```python
from build123d import *

# Parameters (mm, degrees)
SKETCH_1_R                  = 2.25
SKETCH_1_R_2                = 4
EXTRUDE_1_DEPTH             = 2
SKETCH_3_R                  = 0.55
CUT_EXTRUDE_1_DEPTH         = 2
PATTERN_LINEAR_1_COUNT      = 2
PATTERN_LINEAR_1_PITCH      = 2
PATTERN_LINEAR_1_COUNT_DIR2 = 12
PATTERN_LINEAR_1_PITCH_DIR2 = 2.54
SKETCH_4_R                  = 0.9
CUT_EXTRUDE_2_DEPTH         = 2
SKETCH_5_R                  = 0.9
CUT_EXTRUDE_3_DEPTH         = 10
SKETCH_6_R                  = 7.5
SKETCH_6_R_2                = 2.5
SKETCH_6_W                  = 15
SKETCH_6_H                  = 28
SKETCH_6_W_2                = 29
SKETCH_6_H_2                = 5
EXTRUDE_2_DEPTH             = 10
SKETCH_7_W                  = 15
SKETCH_7_H                  = 28
EXTRUDE_3_DEPTH             = 15
SKETCH_8_R                  = 2.5
EXTRUDE_4_DEPTH             = 15.5
SKETCH_9_R                  = 3
EXTRUDE_5_DEPTH             = 5
SKETCH_10_R                 = 3
SKETCH_10_R_2               = 0.3
CUT_EXTRUDE_4_DEPTH         = 4.5
CHAMFER_1_SIZE              = 0.5


with BuildPart() as part:
    # Эскиз1 → Вытянуть1 (new body)
    with BuildSketch(Plane.XY):
        Polygon((10, -60), (65, -60), (65, 60), (-95, 60), (-95, -60), (-20, -60), (-20, -30), (10, -30), align=None)
        with Locations((-90, 55)):
            Circle(SKETCH_1_R, mode=Mode.SUBTRACT)
        with Locations((60, 55)):
            Circle(SKETCH_1_R, mode=Mode.SUBTRACT)
        with Locations((60, -55)):
            Circle(SKETCH_1_R, mode=Mode.SUBTRACT)
        with Locations((-90, -55)):
            Circle(SKETCH_1_R, mode=Mode.SUBTRACT)
        with Locations((-60, 22)):
            Circle(SKETCH_1_R_2, mode=Mode.SUBTRACT)
        with Locations((-30.5, 22)):
            Circle(SKETCH_1_R_2, mode=Mode.SUBTRACT)
        with Locations((-30.5, -23)):
            Circle(SKETCH_1_R_2, mode=Mode.SUBTRACT)
        with Locations((-60, -23)):
            Circle(SKETCH_1_R_2, mode=Mode.SUBTRACT)
        with Locations((24.25, -22.5)):
            Circle(SKETCH_1_R_2, mode=Mode.SUBTRACT)
    extrude(amount=EXTRUDE_1_DEPTH)

    # Эскиз3 → Вырез-Вытянуть1 (cut)
    with BuildSketch(Plane.XY.offset(2)):
        with Locations((-2.25, 7.75)):
            Circle(SKETCH_3_R)
    cut_extrude_1 = extrude(amount=-CUT_EXTRUDE_1_DEPTH, mode=Mode.SUBTRACT)

    # Линейный массив1: Cut-Extrude 1 2 × 12
    with Locations(*[(i * PATTERN_LINEAR_1_PITCH, -j * PATTERN_LINEAR_1_PITCH_DIR2, 0) for i in range(PATTERN_LINEAR_1_COUNT) for j in range(PATTERN_LINEAR_1_COUNT_DIR2) if (i, j) != (0, 0)]):
        add(cut_extrude_1, mode=Mode.SUBTRACT)

    # Эскиз4 → Вырез-Вытянуть2 (cut)
    with BuildSketch(Plane.XY.offset(2)):
        with Locations((17.75, -46.75)):
            Circle(SKETCH_4_R)
        with Locations((-24.75, 16.23)):
            Circle(SKETCH_4_R)
        with Locations((-88.25, 1.58)):
            Circle(SKETCH_4_R)
        with Locations((18, -41.5)):
            Circle(SKETCH_4_R)
        with Locations((14.5, -23.5)):
            Circle(SKETCH_4_R)
        with Locations((18, -36.42)):
            Circle(SKETCH_4_R)
        with Locations((-22.75, 16.23)):
            Circle(SKETCH_4_R)
        with Locations((-4.75, 16.23)):
            Circle(SKETCH_4_R)
        with Locations((18, -31.34)):
            Circle(SKETCH_4_R)
        with Locations((-88.25, -3.5)):
            Circle(SKETCH_4_R)
    extrude(amount=-CUT_EXTRUDE_2_DEPTH, mode=Mode.SUBTRACT)

    # Эскиз5 → Вырез-Вытянуть3 (cut)
    with BuildSketch(Plane.XY.offset(2)):
        with Locations((41.75, 35.75)):
            Circle(SKETCH_5_R)
        with Locations((51.75, 35.75)):
            Circle(SKETCH_5_R)
        with Locations((6.75, 42)):
            Circle(SKETCH_5_R)
        with Locations((16.75, 42)):
            Circle(SKETCH_5_R)
        with Locations((41.75, -35.5)):
            Circle(SKETCH_5_R)
        with Locations((51.75, -35.5)):
            Circle(SKETCH_5_R)
        with Locations((41.75, 0.25)):
            Circle(SKETCH_5_R)
        with Locations((51.75, 0.25)):
            Circle(SKETCH_5_R)
        with Locations((12.25, -55)):
            Circle(SKETCH_5_R)
        with Locations((-79, 56.25)):
            Circle(SKETCH_5_R)
        with Locations(Location((-79, -56.5, 0), (0, 0, 180))):
            Circle(SKETCH_5_R)
        with Locations((8.75, 18.5)):
            Circle(SKETCH_5_R)
        with Locations((16.5, -8)):
            Circle(SKETCH_5_R)
        with Locations((7.75, -22.5)):
            Circle(SKETCH_5_R)
    extrude(amount=-CUT_EXTRUDE_3_DEPTH, mode=Mode.SUBTRACT)

    # Эскиз6 → Вытянуть2 (add)
    # profile 1 of 4: a face of its own
    with BuildSketch(Plane.XY.offset(2)):
        with Locations(Location((-14.5, 1.75, 0), (0, 0, 180))):
            Circle(SKETCH_6_R)
        with Locations((-14.5, 1.75)):
            Circle(SKETCH_6_R_2, mode=Mode.SUBTRACT)
    # profile 2 of 4: a face of its own
    with BuildSketch(Plane.XY.offset(2)):
        with Locations((-69.2, 0)):
            Rectangle(SKETCH_6_W, SKETCH_6_H)
    # profile 3 of 4: a face of its own
    with BuildSketch(Plane.XY.offset(2)):
        with Locations((-41.5, 6.5)):
            Rectangle(SKETCH_6_W_2, SKETCH_6_H_2)
    # profile 4 of 4: a face of its own
    with BuildSketch(Plane.XY.offset(2)):
        with Locations((-41.5, -8.5)):
            Rectangle(SKETCH_6_W_2, SKETCH_6_H_2)
    extrude(amount=EXTRUDE_2_DEPTH)

    # Эскиз7 → Вытянуть3 (add)
    with BuildSketch(Plane.XY.offset(12)):
        with Locations((-69.2, 0)):
            Rectangle(SKETCH_7_W, SKETCH_7_H)
    extrude(amount=EXTRUDE_3_DEPTH)

    # Эскиз8 → Вытянуть4 (add)
    with BuildSketch(Plane.XY.offset(2)):
        with Locations((-8.5, -18)):
            Circle(SKETCH_8_R)
    extrude(amount=-EXTRUDE_4_DEPTH)

    # Эскиз9 → Вытянуть5 (add)
    with BuildSketch(Plane(origin=(0, 0, 0), x_dir=(-1, 0, 0), z_dir=(0, 0, -1))):
        with Locations((8.5, -18)):
            Circle(SKETCH_9_R)
    extrude(amount=EXTRUDE_5_DEPTH)

    # Эскиз10 → Вырез-Вытянуть4 (cut)
    with BuildSketch(Plane.XY):
        with Locations((-8.5, -18)):
            Circle(SKETCH_10_R)
        with Locations((-8.5, -16.496281754)):
            Circle(SKETCH_10_R_2, mode=Mode.SUBTRACT)
        with Locations((-9.77, -19.036281754)):
            Circle(SKETCH_10_R_2, mode=Mode.SUBTRACT)
        with Locations((-7.23, -19.036281754)):
            Circle(SKETCH_10_R_2, mode=Mode.SUBTRACT)
    extrude(amount=-CUT_EXTRUDE_4_DEPTH, mode=Mode.SUBTRACT)

    # Фаска1
    chamfer_1_edges = [part.edges().sort_by_distance(p)[0] for p in [
        (-11, -18, -13.5),
    ]]
    chamfer(chamfer_1_edges, length=CHAMFER_1_SIZE)


solid = part.part
```
The model under review builds one solid part; all positions refer to its coordinate system, in mm. A direction names the side the tool comes from. Coordinates: 2 decimals unless noted, no trailing zeros. Write each loop counter-clockwise with the first axis right and the second up, starting at its lowest first coordinate (ties: lowest second). Pieces come first, ordered by that corner, then holes. Notation, with made-up numbers: (-4, 34.5) - (16, 34.5) arc R16 cw to (16, 42.5) - close; hole circle Ø7 at (54.25, 66.5). An arc over 180 degrees is marked (long way). Write item = value, one per line.
(1) For P1, Ø1.8, axis at x = -0.25, y = -10.03, coming from the -Z side; P2, Ø1.5, axis at y = 6.5, z = 4.5, coming from the -X side; P3, Ø6, axis at x = -90, y = 55, coming from the +Z side, all flat-tipped, find the tip position at first contact; note any pin that passes through.
Result sheet:
P1 = 0
P2 = -76.7
P3 = 2
(2) Machinability: for faces 5 (the face through (-42, -11, 7)), 6 (the face through (-27, 6, 7)), 7 (the face through (-69, 14, 14)), 8 (the face through (-42, 4, 7)), which of the approach directions +Z, -Z, +X, -X, +Y, -Y give a long, thin tool a straight path to every point of the face, cutting with its end or side? Answer none if there is none.
Result sheet:
face_5 = +Z, +X, -Y
face_6 = +Z, +Y, -Y
face_7 = +Z, +X, -X, +Y
face_8 = +Z
(3) For line 1 (Y direction, x = -30, z = 1); line 2 (X direction, y = -46.75, z = 1); line 3 (X direction, y = 42, z = 1), list the stretches that pass through material, from the lowest coordinate up. Write a range as [from, to].
Result sheet:
line_1 = [-60, -26.97], [-19.03, 18.03], [25.97, 60]
line_2 = [-95, -20], [10, 16.85], [18.65, 65]
line_3 = [-95, 5.85], [7.65, 15.85], [17.65, 65]
(4) Mouldability with a two-part tool opening along X and no side actions: class faces 1 (the face through (-56, -9, 7)), 2 (the face through (-27, -9, 7)), 3 (the face through (-9.884, -20.662, -4.746)), 4 (the face through (-42, -8, 12)) as pulls with the +X half, pulls with the -X half, needs draft (parallel to the pull), parting line crosses it, or undercut.
Result sheet:
face_1 = undercut
face_2 = pulls with the +X half
face_3 = parting line crosses it
face_4 = needs draft
(5) Consider section A-A, the plane z = 6. Give the boundary of the cut face in (x, y).
Result sheet:
outline = (-76.7, -14) - (-61.7, -14) - (-61.7, 14) - (-76.7, 14) - close; (-56, -11) - (-27, -11) - (-27, -6) - (-56, -6) - close; (-56, 4) - (-27, 4) - (-27, 9) - (-56, 9) - close; circle Ø15 at (-14.5, 1.75); hole circle Ø5 at (-14.5, 1.75)
(6) Consider section C-C, the plane x = -51. Give the boundary of the cut face in (y, z), then the cut area to 3 significant figures.
Result sheet:
outline = (-60, 0) - (60, 0) - (60, 2) - (9, 2) - (9, 12) - (4, 12) - (4, 2) - (-6, 2) - (-6, 12) - (-11, 12) - (-11, 2) - (-60, 2) - close
area = 340 mm^2
(7) Consider section D-D, the plane z = 19. Give the boundary of the cut face in (x, y), then the cut area to 3 significant figures.
Result sheet:
outline = (-76.7, -14) - (-61.7, -14) - (-61.7, 14) - (-76.7, 14) - close
area = 420 mm^2
(8) Consider section B-B, the plane y = 24. Give the boundary of the cut face in (x, z), then the cut area to 3 significant figures.
Result sheet:
outline = (-95, 0) - (-63.46, 0) - (-63.46, 2) - (-95, 2) - close; (-56.54, 0) - (-33.96, 0) - (-33.96, 2) - (-56.54, 2) - close; (-27.04, 0) - (65, 0) - (65, 2) - (-27.04, 2) - close
area = 292 mm^2
